Design review of the part shown in the three views and the two pictorial views. Dimensions are in mm from the part's minimum x, y and z. A direction names the side the tool comes from. Coordinates: 2 decimals unless noted, no trailing zeros. Order: outer loops, then holes, each group sorted by start corner. A loop starts at its lowest first (then second) coordinate and runs counter-clockwise, first axis right, second up. Notation, with made-up numbers: (-15, 23) - (15, 23) arc R17 cw to (15, 50) - close; hole circle Ø8 at (50, 78). An arc over 180 degrees is marked (long way). One line per item, written item: value. Start each with the question number.
(1) Mouldability with a two-part tool opening along X and no side actions: class the marked faces 4, 5 and 6 as released by +X, released by -X, zero draft, split by the parting line, or undercut.
(2) Consider section D-D on x = 12. Write out the cut boundary in (y, z) (1 decimal).
(3) Consider section B-B on z = 2.5. Write out the cut boundary in (x, y) (1 decimal).
(4) Clearance check with flat-ended pins moving along their axes: pin 1 (2 mm diameter, centred on y = 7, z = 0.5, fed in from +X); pin 2 (1 mm diameter, centred on y = 7.5, z = 1, fed in from -X). State where each tip first meets the part, or that it passes through.
(5) To check wall thickness, follow line 1 along X through (y, z) = (4.75, 3.75) (1 decimal); line 2 along X through (y, z) = (6, 1.5); line 3 along Y through (x, z) = (12.25, 5) (1 decimal). State the ranges of each line that lie inside material, in increasing order.
(6) For the marked faces 1, 2 and 3, list the 3-axis set-ups (+Z, -Z, +X, -X, +Y, -Y) from which the entire face can be reached by the end or side of a thin tool; tool diameter is ignored.
(7) Consider section C-C on y = 7.25. Write out the cut boundary in (x, z) (1 decimal), then the cut area to 3 significant figures.
(8) Consider section A-A on y = 1.5. Write out the cut boundary in (x, z) (1 decimal).
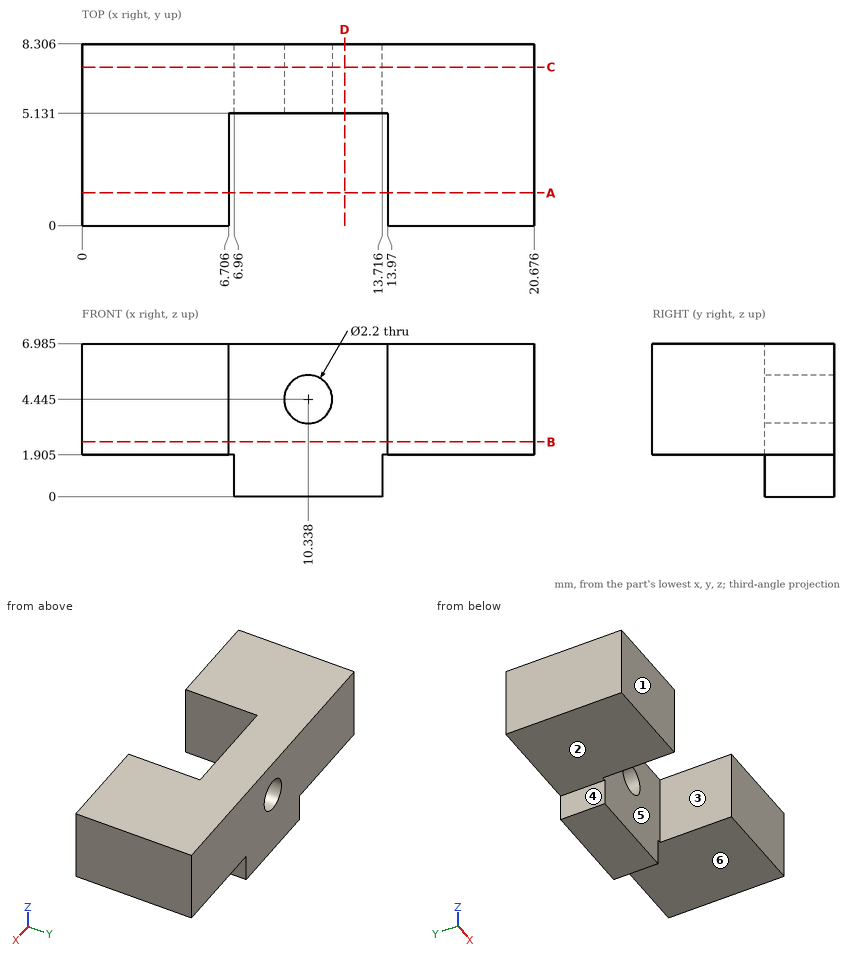
Geometry check:
1. face 4: released by -X
1. face 5: undercut
1. face 6: zero draft
2. outline: (5.1, 0) - (8.3, 0) - (8.3, 7) - (5.1, 7) - close
3. outline: (0, 0) - (6.7, 0) - (6.7, 5.1) - (14, 5.1) - (14, 0) - (20.7, 0) - (20.7, 8.3) - (0, 8.3) - close
4. pin 1: stops at x = 13.72
4. pin 2: stops at x = 6.96
5. line 1: x = 0 to 6.7, 14 to 20.7
5. line 2: x = 6.96 to 13.72
5. line 3: y = 5.1 to 8.3
6. face 1: +Z, -Z, +X, -X, -Y
6. face 2: -Z, -X, +Y, -Y
6. face 3: +Z, -Z, -Y
7. outline: (0, 1.9) - (7, 1.9) - (7, 0) - (13.7, 0) - (13.7, 1.9) - (20.7, 1.9) - (20.7, 7) - (0, 7) - close; hole circle Ø2.2 at (10.3, 4.4)
7. area: 114 mm^2
8. outline: (0, 1.9) - (6.7, 1.9) - (6.7, 7) - (0, 7) - close; (14, 1.9) - (20.7, 1.9) - (20.7, 7) - (14, 7) - close
